Part print with two shaded views. Sizes in mm from the minimum x, y, z corner. A direction names the side the tool comes from. Give positions to 0.01 mm unless a question says otherwise; leave off trailing zeros. Order: outer loops, then holes, each group sorted by start corner. A loop starts at its lowest first (then second) coordinate and runs counter-clockwise, first axis right, second up. Notation, with made-up numbers: M 24.5,-10.75 L 54.5,-10.75 A14 cw 54.5,-1.75 Z; hole C 49.5,88 d3. An arc over 180 degrees is marked long. Return JSON: item names as keys, results as strings. Group by question number.
1. Wall check: probe 1 along X at (y, z) = (77, 240); probe 2 along Y at (x, z) = (34, 32); probe 3 along Z at (x, y) = (43, 5.5). Give the ranges that are in metal, low to high. Write a range as [from, to].
2. Slice it at B-B on y = 81.5. List the corners of the cut face in (x, z), then the cut area to 3 significant figures.
3. Slice it at D-D on z = 37. List the corners of the cut face in (x, y).
4. Slice it at A-A on x = 50. List the corners of the cut face in (y, z), then the cut area to 4 significant figures.
5. 3-axis set-ups, long thin cutter, end or side, ignore diameter. For the marked faces 1 and 2: which of +Z, -Z, +X, -X, +Y, -Y reach the whole face in a straight line?
6. Slice it at C-C on x = 20. List the corners of the cut face in (y, z), then the cut area to 3 significant figures.
7. Pin check, flat tips, straight feed: pin 1 (12 mm diameter, centred on x = 87, y = 88, fed in from -Z); pin 2 (12 mm diameter, centred on x = 53, z = 48.5, fed in from -Y); pin 3 (8 mm diameter, centred on y = 95, z = 51.5, fed in from -X). Stop position of each tip, or through.
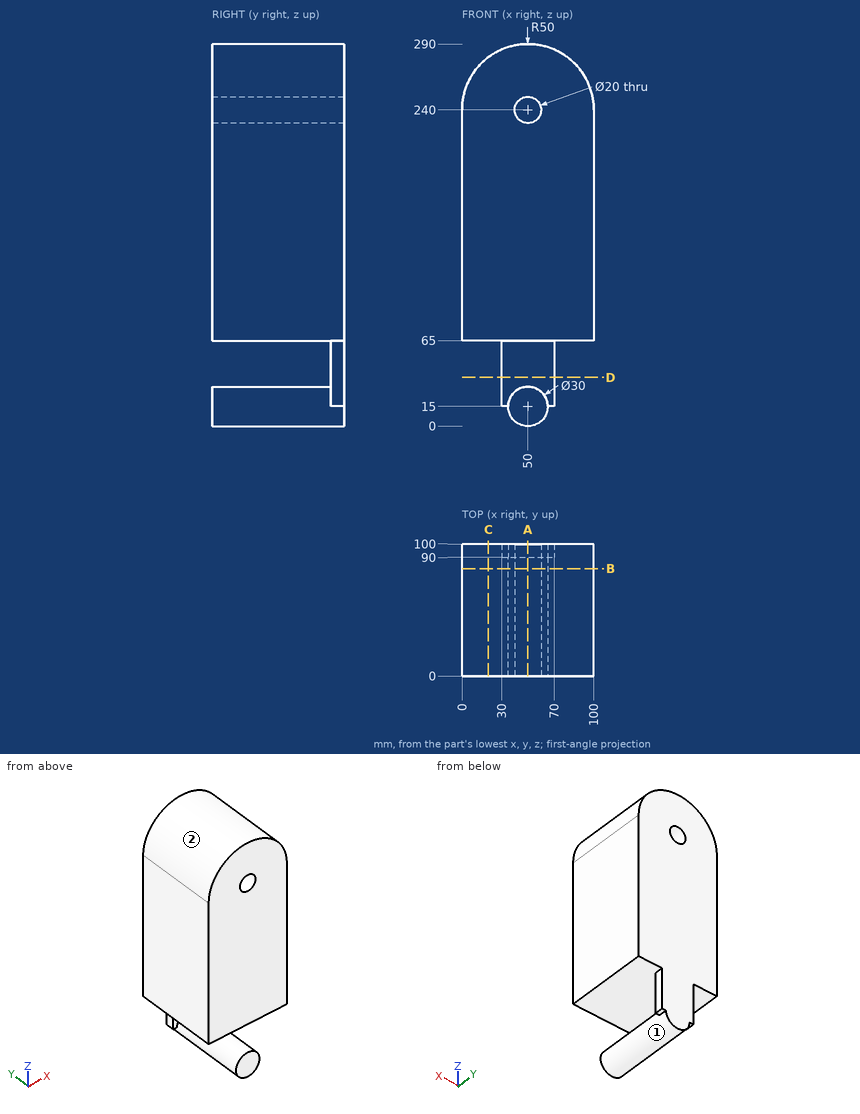
Result:
{
 "1": {"probe 1": "x = [0, 40], [60, 100]", "probe 2": "y = [90, 100]", "probe 3": "z = [1.73, 28.27], [65, 232.86], [247.14, 289.51]"},
 "2": {"outline": "M 0,65 L 100,65 L 100,240 A50 ccw 0,240 Z; C 50,15 d30; hole C 50,240 d20", "area": "21,800 mm2"},
 "3": {"outline": "M 30,90 L 70,90 L 70,100 L 30,100 Z"},
 "4": {"outline": "M 0,0 L 100,0 L 100,230 L 0,230 L 0,65 L 90,65 L 90,30 L 0,30 Z; M 0,250 L 100,250 L 100,290 L 0,290 Z", "area": "23,850 mm2"},
 "5": {"face 1": "-Y", "face 2": "+Z, +Y, -Y"},
 "6": {"outline": "M 0,65 L 100,65 L 100,280 L 0,280 Z", "area": "21,500 mm2"},
 "7": {"pin 1": "stops at z = 65", "pin 2": "stops at y = 90", "pin 3": "stops at x = 30"}
}
